from build123d import *

# Parameters (mm, degrees)
F0_W      = 86
F0_H      = 75
F0_W_2    = 84.1
F0_H_2    = 55.1
F1_DEPTH  = 45
F2_W      = 86
F2_H      = 75
F2_W_2    = 84.1
F2_H_2    = 55.1
F3_DEPTH  = 5
F4_W      = 25
F4_H      = 20
F4_W_2    = 46
F5_DEPTH  = 25
F6_R      = 2.75
F7_DEPTH  = 50.001
F8_R      = 5
F9_R      = 2.75
F9_R_2    = 4.275
F9_R_3    = 4.25
F10_DEPTH = 2.5
F11_R     = 4.275
F11_R_2   = 4.25
F12_DEPTH = 2.5


with BuildPart() as f1:
    # F0 (on Top) → F1 (new body)
    with BuildSketch(Plane.XY):
        Rectangle(F0_W, F0_H)
        Rectangle(F0_W_2, F0_H_2, mode=Mode.SUBTRACT)
    extrude(amount=F1_DEPTH)

    # F2 (on face) → F3 (join)
    with BuildSketch(Plane.XY.offset(45)):
        Rectangle(F2_W, F2_H)
        Rectangle(F2_W_2, F2_H_2, mode=Mode.SUBTRACT)
        Rectangle(F2_W_2, F2_H_2)
    extrude(amount=F3_DEPTH)

    # F4 (on face) → F5 (cut)
    with BuildSketch(Plane.XZ.offset(37.5)):
        with Locations((-24.55, 35)):
            Rectangle(F4_W, F4_H)
        with Locations((12.95, 35)):
            Rectangle(F4_W_2, F4_H)
    extrude(amount=-F5_DEPTH, mode=Mode.SUBTRACT)

    # F6 (on face) → F7 (cut, through all)
    with BuildSketch(Plane(origin=(0, 0, 0), x_dir=(1, 0, 0), z_dir=(0, 0, -1))):
        with Locations((-38.025, 32.525)):
            Circle(F6_R)
        with Locations((0, 32.525)):
            Circle(F6_R)
        with Locations((38.025, 32.525)):
            Circle(F6_R)
        with Locations((38.025, -32.525)):
            Circle(F6_R)
        with Locations((0, -32.525)):
            Circle(F6_R)
        with Locations((-38.025, -32.525)):
            Circle(F6_R)
    extrude(amount=-F7_DEPTH, mode=Mode.SUBTRACT)

    # F8
    f8_edges = [f1.edges().sort_by_distance(p)[0] for p in [
        (43, -37.5, 25),
        (43, 37.5, 25),
        (-43, 37.5, 25),
        (-43, -37.5, 25),
    ]]
    fillet(f8_edges, radius=F8_R)

    # F9 (on face) → F10 (cut)
    with BuildSketch(Plane.XY.offset(50)):
        with BuildLine():
            Line((-38, -37.5), (-33.75, -37.5))
            Line((-33.75, -37.5), (-33.75, -32.5))
            ThreePointArc((-33.75, -32.5), (-41.00520382, -35.50520382), (-38, -28.25))
            Line((-38, -28.25), (-43, -28.25))
            Line((-43, -28.25), (-43, -32.5))
            ThreePointArc((-43, -32.5), (-41.5355339059, -36.0355339059), (-38, -37.5))
        make_face()
        with BuildLine():
            ThreePointArc((-38, -28.25), (-41.00520382, -35.50520382), (-33.75, -32.5))
            ThreePointArc((-33.75, -32.5), (-34.99479618, -29.49479618), (-38, -28.25))
        make_face()
        with Locations((-38.025, -32.525)):
            Circle(F9_R, mode=Mode.SUBTRACT)
        with Locations((0, -32.525)):
            Circle(F9_R_2)
        with Locations((0, -32.525)):
            Circle(F9_R, mode=Mode.SUBTRACT)
        with BuildLine():
            ThreePointArc((38, -37.5), (41.5355339059, -36.0355339059), (43, -32.5))
            Line((43, -32.5), (43, -28.25))
            Line((43, -28.25), (38, -28.25))
            ThreePointArc((38, -28.25), (41.00520382, -29.49479618), (42.25, -32.5))
            ThreePointArc((42.25, -32.5), (38, -36.75), (33.75, -32.5))
            Line((33.75, -32.5), (33.75, -37.5))
            Line((33.75, -37.5), (38, -37.5))
        make_face()
        with BuildLine():
            ThreePointArc((42.25, -32.5), (41.00520382, -29.49479618), (38, -28.25))
            ThreePointArc((38, -28.25), (34.99479618, -29.49479618), (33.75, -32.5))
            ThreePointArc((33.75, -32.5), (38, -36.75), (42.25, -32.5))
        make_face()
        with Locations((38.025, -32.525)):
            Circle(F9_R, mode=Mode.SUBTRACT)
        with Locations((0, 32.525)):
            Circle(F9_R_3)
        with Locations((0, 32.525)):
            Circle(F9_R, mode=Mode.SUBTRACT)
        with BuildLine():
            Line((-33.75, 32.5), (-33.75, 37.5))
            Line((-33.75, 37.5), (-38, 37.5))
            ThreePointArc((-38, 37.5), (-41.5355339059, 36.0355339059), (-43, 32.5))
            Line((-43, 32.5), (-43, 28.25))
            Line((-43, 28.25), (-38, 28.25))
            ThreePointArc((-38, 28.25), (-41.00520382, 35.50520382), (-33.75, 32.5))
        make_face()
        with BuildLine():
            ThreePointArc((-38, 28.25), (-34.99479618, 29.49479618), (-33.75, 32.5))
            ThreePointArc((-33.75, 32.5), (-41.00520382, 35.50520382), (-38, 28.25))
        make_face()
        with Locations((-38.025, 32.525)):
            Circle(F9_R, mode=Mode.SUBTRACT)
        with BuildLine():
            Line((38, 28.25), (43, 28.25))
            Line((43, 28.25), (43, 32.5))
            ThreePointArc((43, 32.5), (41.5355339059, 36.0355339059), (38, 37.5))
            Line((38, 37.5), (33.75, 37.5))
            Line((33.75, 37.5), (33.75, 32.5))
            ThreePointArc((33.75, 32.5), (38, 36.75), (42.25, 32.5))
            ThreePointArc((42.25, 32.5), (41.00520382, 29.49479618), (38, 28.25))
        make_face()
        with BuildLine():
            ThreePointArc((33.75, 32.5), (34.99479618, 29.49479618), (38, 28.25))
            ThreePointArc((38, 28.25), (41.00520382, 29.49479618), (42.25, 32.5))
            ThreePointArc((42.25, 32.5), (38, 36.75), (33.75, 32.5))
        make_face()
        with Locations((38.025, 32.525)):
            Circle(F9_R, mode=Mode.SUBTRACT)
    extrude(amount=-F10_DEPTH, mode=Mode.SUBTRACT)

    # F11 (on face) → F12 (join)
    with BuildSketch(Plane.XY.offset(50)):
        with BuildLine():
            Line((43, 28.25), (38, 28.25))
            ThreePointArc((38, 28.25), (34.99479618, 29.49479618), (33.75, 32.5))
            Line((33.75, 32.5), (33.75, 37.5))
            Line((33.75, 37.5), (-33.75, 37.5))
            Line((-33.75, 37.5), (-33.75, 32.5))
            ThreePointArc((-33.75, 32.5), (-34.99479618, 29.49479618), (-38, 28.25))
            Line((-38, 28.25), (-43, 28.25))
            Line((-43, 28.25), (-43, -28.25))
            Line((-43, -28.25), (-38, -28.25))
            ThreePointArc((-38, -28.25), (-34.99479618, -29.49479618), (-33.75, -32.5))
            Line((-33.75, -32.5), (-33.75, -37.5))
            Line((-33.75, -37.5), (33.75, -37.5))
            Line((33.75, -37.5), (33.75, -32.5))
            ThreePointArc((33.75, -32.5), (34.99479618, -29.49479618), (38, -28.25))
            Line((38, -28.25), (43, -28.25))
            Line((43, -28.25), (43, 28.25))
        make_face()
        with Locations((0, -32.525)):
            Circle(F11_R, mode=Mode.SUBTRACT)
        with Locations((0, 32.525)):
            Circle(F11_R_2, mode=Mode.SUBTRACT)
    extrude(amount=F12_DEPTH)


solid = f1.part
Could you check a few things on this model? Use its own coordinates, in mm. A direction names the side the tool comes from. Coordinates: 2 decimals unless noted, no trailing zeros. Loops run counter-clockwise (first coordinate to the right, second up) from the corner with the lowest first, then second, coordinate; pieces in that order, holes last.
1. Imagine slicing it at B-B (z = 31.5). Please give me the cut outline in (x, y) (3 decimals).
2. For faces 1 (the face through (33.75, 35, 50)), 2 (the face through (-1, -27.55, 17)), 3 (the face through (33.75, -35, 50)), 4 (the face through (-25, -33, 25)), which set-ups out of +Z, -Z, +X, -X, +Y, -Y let a thin tool reach every point of the face, with its end or its side?
3. Imagine slicing it at D-D (z = 10.5). Please give me the cut outline in (x, y) (3 decimals), and give its area (3 significant figures).
4. I need wall thicknesses on L1, parallel to X at y = -32.5, z = 21.5; L2, parallel to X at y = -12, z = 41; L3, parallel to Y at x = -5.5, z = 12. Which ranges of each line are inside material? Lowest first, please.
5. We'd pull the mould along Y, two halves only. Please class faces 5 (the face through (-37.05, -29, 35)), 6 (the face through (34.96, -29.53, 49.96)), 7 (the face through (-0.6, -29.84, 46.23)), 8 (the face through (-42.05, 0, 22)): released by +Y, released by -Y, zero draft, split by the parting line, or undercut.
6. Imagine slicing it at C-C (x = -9). Please give me the cut outline in (y, z), and give its area (3 significant figures).
7. Imagine slicing it at A-A (x = 0). Give the number of separate pieces and of enclosed holes in the cut face, and give its area (3 significant figures).
8. For P1, Ø4, axis at x = 16.5, y = -15.5, coming from the -Z side; P2, Ø2.5, axis at y = -34, z = 51, coming from the +X side; P3, Ø4.5, axis at x = 38, y = -31, coming from the +Z side, each with a flat end and sliding along its axis, tell me the tip position at first contact or that it passes through.
Computed values:
1. outline: (-43, -32.5) arc R5 ccw to (-38, -37.5) - (-37.05, -37.5) - (-37.05, -35.096) arc R2.75 cw (long way) to (-37.05, -29.954) - (-37.05, -27.55) - (-42.05, -27.55) - (-42.05, 27.55) - (42.05, 27.55) - (42.05, -27.55) - (35.95, -27.55) - (35.95, -30.72) arc R2.75 cw (long way) to (35.95, -34.33) - (35.95, -37.5) - (38, -37.5) arc R5 ccw to (43, -32.5) - (43, 32.5) arc R5 ccw to (38, 37.5) - (-38, 37.5) arc R5 ccw to (-43, 32.5) - close; (-12.05, -37.5) - (-10.05, -37.5) - (-10.05, -27.55) - (-12.05, -27.55) - close; hole circle Ø5.5 at (-38.025, 32.525); hole circle Ø5.5 at (0, 32.525); hole circle Ø5.5 at (38.025, 32.525)
2. face 1: +Z, +X, +Y
2. face 2: -Z
2. face 3: +Z, +X, -Y
2. face 4: -Y
3. outline: (-43, -32.5) arc R5 ccw to (-38, -37.5) - (38, -37.5) arc R5 ccw to (43, -32.5) - (43, 32.5) arc R5 ccw to (38, 37.5) - (-38, 37.5) arc R5 ccw to (-43, 32.5) - close; hole (-42.05, -27.55) - (42.05, -27.55) - (42.05, 27.55) - (-42.05, 27.55) - close; hole circle Ø5.5 at (-38.025, -32.525); hole circle Ø5.5 at (-38.025, 32.525); hole circle Ø5.5 at (0, -32.525); hole circle Ø5.5 at (0, 32.525); hole circle Ø5.5 at (38.025, -32.525); hole circle Ø5.5 at (38.025, 32.525)
3. area: 1,650 mm2
4. L1: x = -43 to -40.77, -35.28 to -2.75, 2.75 to 35.28, 40.77 to 43
4. L2: x = -43 to -42.05, 42.05 to 43
4. L3: y = -37.5 to -27.55, 27.55 to 37.5
5. face 5: zero draft
5. face 6: released by -Y
5. face 7: undercut
5. face 8: undercut
6. outline: (-37.5, 0) - (-27.55, 0) - (-27.55, 25) - (-37.5, 25) - close; (-37.5, 45) - (27.55, 45) - (27.55, 0) - (37.5, 0) - (37.5, 52.5) - (-37.5, 52.5) - close
6. area: 1,260 mm2
7. separate pieces: 5
7. enclosed holes: 0
7. area: 761 mm2
8. P1: stops at z = 45
8. P2: stops at x = 33.75
8. P3: stops at z = 47.5
